from build123d import *

# Parameters (mm, degrees)
SKETCH_2_W               = 265
SKETCH_2_H               = 265
SKETCH_2_R               = 10
EXTRUDE_585_DEPTH        = 3
CUT_EXTRUDE_2_DEPTH      = 188.407310423
CUT_EXTRUDE_2_DEPTH_BACK = 188.407310423
SKETCH_3_R               = 25
SKETCH_3_R_2             = 1.75
FILLET_2_R               = 10


with BuildPart() as part:
    # 草图2 → Extrude 585 (new body)
    with BuildSketch(Plane(origin=(0, 0, 0), x_dir=(1, 0, 0), z_dir=(0, 1, 0))):
        Rectangle(SKETCH_2_W, SKETCH_2_H)
        with Locations(Location((0, 0, 0), (0, 0, 270))):
            Circle(SKETCH_2_R, mode=Mode.SUBTRACT)
    extrude(amount=EXTRUDE_585_DEPTH)

    # 草图3 → 切除-拉伸2 (cut, two sides: drawn at the far end of the back side and taken through both)
    with BuildSketch(Plane(origin=(0, 3, 0), x_dir=(1, 0, 0), z_dir=(0, 1, 0)).offset(-CUT_EXTRUDE_2_DEPTH_BACK)):
        with Locations((-132.5, -132.5)):
            Circle(SKETCH_3_R)
        with Locations((-132.5, 132.5)):
            Circle(SKETCH_3_R)
        with Locations(Location((-124.5, 101, 0), (0, 0, 270))):
            Circle(SKETCH_3_R_2)
        with Locations(Location((-101, 124.5, 0), (0, 0, 270))):
            Circle(SKETCH_3_R_2)
        with Locations(Location((-124.5, -101, 0), (0, 0, 270))):
            Circle(SKETCH_3_R_2)
        with Locations(Location((-101, -124.5, 0), (0, 0, 270))):
            Circle(SKETCH_3_R_2)
        with Locations((132.5, 132.5)):
            Circle(SKETCH_3_R)
        with Locations(Location((101, 124.5, 0), (0, 0, 270))):
            Circle(SKETCH_3_R_2)
        with Locations(Location((124.5, 101, 0), (0, 0, 270))):
            Circle(SKETCH_3_R_2)
        with Locations((132.5, -132.5)):
            Circle(SKETCH_3_R)
        with Locations(Location((124.5, -101, 0), (0, 0, 270))):
            Circle(SKETCH_3_R_2)
        with Locations(Location((101, -124.5, 0), (0, 0, 270))):
            Circle(SKETCH_3_R_2)
    extrude(amount=CUT_EXTRUDE_2_DEPTH + CUT_EXTRUDE_2_DEPTH_BACK, mode=Mode.SUBTRACT)

    # 圆角2
    fillet_2_edges = [part.edges().sort_by_distance(p)[0] for p in [
        (132.5, 1.5, -107.5),
        (107.5, 1.5, -132.5),
        (-107.5, 1.5, -132.5),
        (-132.5, 1.5, -107.5),
        (107.5, 1.5, 132.5),
        (132.5, 1.5, 107.5),
        (-107.5, 1.5, 132.5),
        (-132.5, 1.5, 107.5),
    ]]
    fillet(fillet_2_edges, radius=FILLET_2_R)


solid = part.part
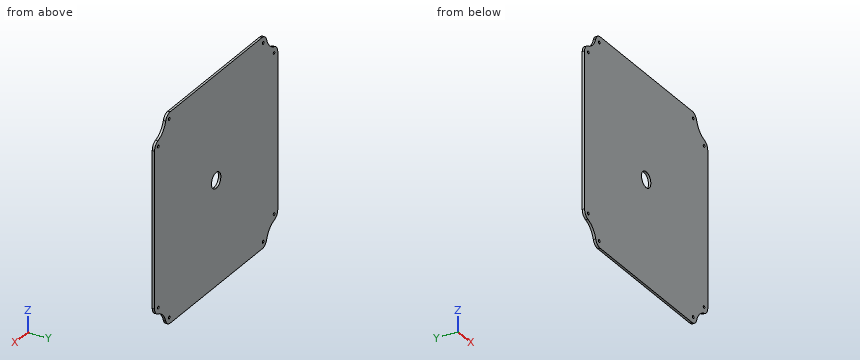
Read the model definition and answer for the solid it produces. Units are mm, in the model's axes. Coordinates: 2 decimals unless noted, no trailing zeros. Write each loop counter-clockwise with the first axis right and the second up, starting at its lowest first coordinate (ties: lowest second). Pieces come first, ordered by that corner, then holes. Notation, with made-up numbers: M 40,87.5 L 92,87.5 A33 ccw 92,123.5 Z; hole C -32,-36.75 d2. An arc over 180 degrees is marked long. Use a Markdown table: item, result.
Q1. This flat-tipped pin is pushed along its axis until it touches: pin 1 Ø2 at (x, z) = (2.5, -71) entering from -Y. Where does it stop, or does it pass through?
Answer block:
| item | result |
|---|---|
| pin 1 | stops at y = 0 |
Q2. The part is cut by section B-B, the plane x = -6. Write down the section's boundary in (y, z), then the cut area to 3 significant figures.
Answer block:
| item | result |
|---|---|
| outline | M 0,-132.5 L 3,-132.5 L 3,-8 L 0,-8 Z; M 0,8 L 3,8 L 3,132.5 L 0,132.5 Z |
| area | 747 mm2 |
Q3. Straight lines are drawn through the part: L1, parallel to X at y = 0.9, z = -124.5; L2, parallel to Z at x = -101, y = 2.2. For each, find the intervals that lie inside material, in ascending order. Write a range as [from, to].
Answer block:
| item | result |
|---|---|
| L1 | x = [-108.81, -102.75], [-99.25, 99.25], [102.75, 108.81] |
| L2 | z = [-132.29, -126.25], [-122.75, 122.75], [126.25, 132.29] |
Q4. The part is cut by section A-A, the plane y = 1.85. Give the number of separate pieces and of enclosed holes in the cut face, then the cut area to 3 significant figures.
Answer block:
| item | result |
|---|---|
| separate pieces | 1 |
| enclosed holes | 9 |
| area | 67,800 mm2 |
